from build123d import *

# Parameters (mm, degrees)
SKETCH_1_W          = 54.5
SKETCH_1_H          = 44.5
EXTRUDE_1_DEPTH     = 5
SKETCH_2_W          = 29.5
SKETCH_2_H          = 29.5
CUT_EXTRUDE_1_DEPTH = 71.537224215
FILLET_1_R          = 1.25
SKETCH_4_R          = 1.5
CUT_EXTRUDE_2_DEPTH = 71.537224215
SKETCH_7_R          = 1.5
CUT_EXTRUDE_3_DEPTH = 71.537224215


with BuildPart() as part:
    # Эскиз1 → Бобышка-Вытянуть1 (new body)
    with BuildSketch(Plane(origin=(0, 0, 0), x_dir=(1, 0, 0), z_dir=(0, 1, 0))):
        with Locations((27.25, 22.25)):
            Rectangle(SKETCH_1_W, SKETCH_1_H)
    extrude(amount=EXTRUDE_1_DEPTH)

    # Эскиз2 → Вырез-Вытянуть1 (cut, through all)
    with BuildSketch(Plane(origin=(0, 5, 0), x_dir=(1, 0, 0), z_dir=(0, 1, 0))):
        with Locations((22.25, 22.25)):
            Rectangle(SKETCH_2_W, SKETCH_2_H)
    extrude(amount=-CUT_EXTRUDE_1_DEPTH, mode=Mode.SUBTRACT)

    # Скругление1
    fillet_1_edges = [part.edges().sort_by_distance(p)[0] for p in [
        (7.5, 2.5, -7.5),
        (7.5, 2.5, -37),
        (37, 2.5, -37),
        (37, 2.5, -7.5),
    ]]
    fillet(fillet_1_edges, radius=FILLET_1_R)

    # Эскиз4 → Вырез-Вытянуть2 (cut, through all)
    with BuildSketch(Plane(origin=(0, 5, 0), x_dir=(1, 0, 0), z_dir=(0, 1, 0))):
        with Locations(Location((44.75, 22.25, 0), (0, 0, 270))):
            Circle(SKETCH_4_R)
    extrude(amount=-CUT_EXTRUDE_2_DEPTH, mode=Mode.SUBTRACT)

    # Эскиз7 → Вырез-Вытянуть3 (cut, through all)
    with BuildSketch(Plane.XZ):
        with Locations(Location((6.310660172, -38.189339828, 0), (0, 0, 270))):
            Circle(SKETCH_7_R)
        with Locations(Location((38.189339828, -38.189339828, 0), (0, 0, 270))):
            Circle(SKETCH_7_R)
        with Locations(Location((6.310660172, -6.310660172, 0), (0, 0, 270))):
            Circle(SKETCH_7_R)
        with Locations(Location((38.189339828, -6.310660172, 0), (0, 0, 270))):
            Circle(SKETCH_7_R)
        with Locations(Location((22.25, -39.25, 0), (0, 0, 270))):
            Circle(SKETCH_7_R)
        with Locations(Location((5.25, -22.25, 0), (0, 0, 270))):
            Circle(SKETCH_7_R)
        with Locations(Location((22.25, -5.25, 0), (0, 0, 90))):
            Circle(SKETCH_7_R)
    extrude(amount=-CUT_EXTRUDE_3_DEPTH, mode=Mode.SUBTRACT)


solid = part.part
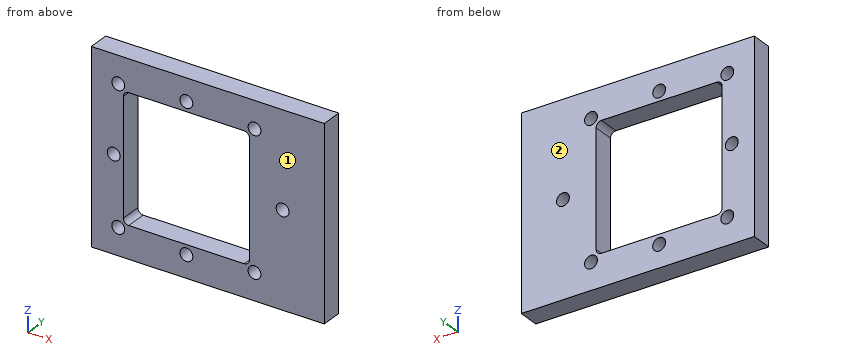
Check sheet for the modelled part. Datum: model origin and axes. Units: mm. Face numbers are marked on the shaded views. Give positions to 0.01 mm unless a question says otherwise; leave off trailing zeros. Write each loop counter-clockwise with the first axis right and the second up, starting at its lowest first coordinate (ties: lowest second). Pieces come first, ordered by that corner, then holes. Notation, with made-up numbers: M 64,25.5 L 107,25.5 A23 ccw 107,40.5 Z; hole C 71.25,-21.75 d6. An arc over 180 degrees is marked long. Use one line per item in the form item = value.
(1) Section check B-B on z = -15. Record the boundary of the cut face in (x, y), plus the area to 3 significant figures.
Answer block:
outline = M 0,0 L 7.5,0 L 7.5,5 L 0,5 Z; M 37,0 L 54.5,0 L 54.5,5 L 37,5 Z
area = 125 mm2
(2) Section check D-D on z = -22.25. Record the boundary of the cut face in (x, y), plus the area to 3 significant figures.
Answer block:
outline = M 0,0 L 3.75,0 L 3.75,5 L 0,5 Z; M 6.75,0 L 7.5,0 L 7.5,5 L 6.75,5 Z; M 37,0 L 43.25,0 L 43.25,5 L 37,5 Z; M 46.25,0 L 54.5,0 L 54.5,5 L 46.25,5 Z
area = 95.0 mm2
(3) Draft check along Y on the marked faces 1 and 2. Enter one of: pulls with the +Y half, pulls with the -Y half, needs draft (parallel to the pull), parting line crosses it, or undercut.
Answer block:
face_1 = pulls with the -Y half
face_2 = pulls with the +Y half
(4) Section check A-A on x = 12.5. Record the boundary of the cut face in (y, z).
Answer block:
outline = M 0,-44.5 L 5,-44.5 L 5,-37 L 0,-37 Z; M 0,-7.5 L 5,-7.5 L 5,0 L 0,0 Z
(5) Section check C-C on x = 22.25. Record the boundary of the cut face in (y, z), plus the area to 3 significant figures.
Answer block:
outline = M 0,-44.5 L 5,-44.5 L 5,-40.75 L 0,-40.75 Z; M 0,-37.75 L 5,-37.75 L 5,-37 L 0,-37 Z; M 0,-7.5 L 5,-7.5 L 5,-6.75 L 0,-6.75 Z; M 0,-3.75 L 5,-3.75 L 5,0 L 0,0 Z
area = 45.0 mm2
(6) Material ranges on line 1 along X through (y, z) = (2.4, -22.25); line 2 along X through (y, z) = (1.2, -33.5); line 3 along Z through (x, y) = (18.5, 1.15), recorded low to high.
Answer block:
line_1 = 0 to 3.75, 6.75 to 7.5, 37 to 43.25, 46.25 to 54.5
line_2 = 0 to 7.5, 37 to 54.5
line_3 = -44.5 to -37, -7.5 to 0
(7) Depth check by flat-ended pin: P1, Ø4, axis at x = 5.25, z = -22.25, coming from the +Y side. Enter the tip coordinate at first touch or a pass-through.
Answer block:
P1 = 5
